Input: part model. Units: mm. Frame: model coordinates. Face numbers are marked on the shaded views. A direction names the side the tool comes from. Give positions to 0.01 mm unless a question says otherwise; leave off trailing zeros. Order: outer loops, then holes, each group sorted by start corner. A loop starts at its lowest first (then second) coordinate and runs counter-clockwise, first axis right, second up. Notation, with made-up numbers: (45.5, -2) - (92.5, -2) arc R17 cw to (92.5, 23) - close; hole circle Ø11 at (58, -29.5). An arc over 180 degrees is marked (long way). Use a Markdown table: item, result.
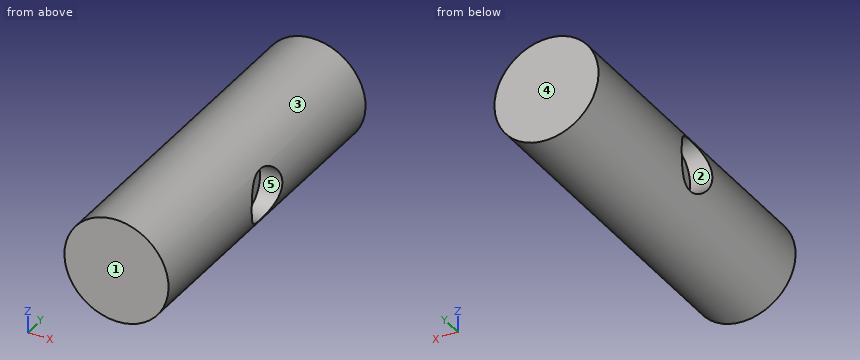
from build123d import *

# Parameters (mm, degrees)
SKETCH_1_R          = 7
EXTRUDE_1_DEPTH     = 45
CUT_EXTRUDE_1_DEPTH = 11
CUT_EXTRUDE_START   = 11
CUT_EXTRUDE_2_DEPTH = 11


with BuildPart() as part:
    # 草图1 → 凸台-拉伸1 (new body)
    with BuildSketch(Plane(origin=(0, 0, 0), x_dir=(1, 0, 0), z_dir=(0, 1, 0))):
        with Locations(Location((0, 0, 0), (0, 0, 90))):
            Circle(SKETCH_1_R)
    extrude(amount=EXTRUDE_1_DEPTH)

    # 草图4 → 切除-拉伸1 (cut)
    with BuildSketch(Plane(origin=(15, 0, 0), x_dir=(0, 0, -1), z_dir=(1, 0, 0))):
        with BuildLine():
            ThreePointArc((3.5, 22.5), (0, 26), (-3.5, 22.5))
            Line((-3.5, 22.5), (3.5, 22.5))
        make_face()
        with BuildLine():
            Line((3.5, 22.5), (-3.5, 22.5))
            ThreePointArc((-3.5, 22.5), (0, 19), (3.5, 22.5))
        make_face()
    extrude(amount=-CUT_EXTRUDE_1_DEPTH, mode=Mode.SUBTRACT)

    # 草图5 → 切除-拉伸2 (cut)
    with BuildSketch(Plane(origin=(-15, 0, 0), x_dir=(0, 0, -1), z_dir=(1, 0, 0)).offset(CUT_EXTRUDE_START)):
        with BuildLine():
            ThreePointArc((-3.5, 22.5), (0, 19), (3.5, 22.5))
            Line((3.5, 22.5), (-3.5, 22.5))
        make_face()
        with BuildLine():
            Line((-3.5, 22.5), (3.5, 22.5))
            ThreePointArc((3.5, 22.5), (0, 26), (-3.5, 22.5))
        make_face()
    extrude(amount=-CUT_EXTRUDE_2_DEPTH, mode=Mode.SUBTRACT)


solid = part.part
1. Section query C-C (x = 5). Return loops of the section in (y, z).
Response:
| item | result |
|---|---|
| outline | (0, -4.9) - (45, -4.9) - (45, 4.9) - (0, 4.9) - close; hole circle Ø7 at (22.5, 0) |
2. Section query B-B (y = 22.5). Return loops of the section in (x, z), then the cut area to 3 significant figures.
Response:
| item | result |
|---|---|
| outline | (-6.06, -3.5) arc R7 ccw to (6.06, -3.5) - (4, -3.5) - (4, 3.5) - (6.06, 3.5) arc R7 ccw to (-6.06, 3.5) - (-4, 3.5) - (-4, -3.5) - close |
| area | 116 mm^2 |
3. Mould query, pull axis Z, two halves, no side actions, for the marked faces 1, 2 and 3. Classes: pulls with the +Z half, pulls with the -Z half, needs draft (parallel to the pull), parting line crosses it, or undercut.
Response:
| item | result |
|---|---|
| face 1 | needs draft |
| face 2 | undercut |
| face 3 | parting line crosses it |
4. Section query A-A (z = -1.25). Return loops of the section in (x, y).
Response:
| item | result |
|---|---|
| outline | (-6.89, 0) - (6.89, 0) - (6.89, 19.23) - (4, 19.23) - (4, 25.77) - (6.89, 25.77) - (6.89, 45) - (-6.89, 45) - (-6.89, 25.77) - (-4, 25.77) - (-4, 19.23) - (-6.89, 19.23) - close |
5. Section query D-D (x = -2). Return loops of the section in (y, z), then the cut area to 3 significant figures.
Response:
| item | result |
|---|---|
| outline | (0, -6.71) - (45, -6.71) - (45, 6.71) - (0, 6.71) - close |
| area | 604 mm^2 |
6. Set-up query: the marked faces 4 and 5. Return all of +Z, -Z, +X, -X, +Y, -Y with unobstructed straight access to the full face (end or side cutting, diameter ignored); none if empty.
Response:
| item | result |
|---|---|
| face 4 | +Z, -Z, +X, -X, +Y |
| face 5 | +X |
7. Material intervals for line 1 along Y through (x, z) = (5.8, 0); line 2 along Y through (x, z) = (-5, -2.25); line 3 along X through (y, z) = (2.5, -0.5), sorted ascending.
Response:
| item | result |
|---|---|
| line 1 | y = 0 to 19, 26 to 45 |
| line 2 | y = 0 to 19.82, 25.18 to 45 |
| line 3 | x = -6.98 to 6.98 |
8. Pin query (flat end, axial travel): pin 1 (6 mm diameter, centred on x = -4, y = 35, fed in from +Z); pin 2 (2 mm diameter, centred on y = 26, z = 4, fed in from +X); pin 3 (1 mm diameter, centred on y = 23, z = 0, fed in from -X). Return the tip coordinate at first contact, or that it passes through.
Response:
| item | result |
|---|---|
| pin 1 | stops at z = 6.93 |
| pin 2 | stops at x = 6.32 |
| pin 3 | stops at x = -4 |
